Autodesk Inventor part; units mm, degrees
ref_plane "YZ Plane" through (0, 0, 0) normal (1, 0, 0) x (0, 1, 0)
ref_plane "XZ Plane" through (0, 0, 0) normal (0, 1, 0) x (-1, 0, 0)
ref_plane "XY Plane" through (0, 0, 0) normal (0, 0, 1) x (1, 0, 0)
sketch "Sketch1" plane through (0, 0, 0) normal (0, 1, 0) x (-1, 0, 0)
  circle A0 centre (0, 0) radius 3.75
  circle A1 centre (0, 0) radius 6
  dimension "d0" = 7.5
  dimension "d1" = 12
extrude "Extrusion1" add sketch "Sketch1" along normal blind 50 contours A0 | A1
extrude "Extrusion2" add sketch "Sketch1" against normal blind 2 contours A0
sketch "Sketch2" plane through (0, -2, 0) normal (0, -1, 0) x (1, 0, 0)
  circle A0 centre (0, 0) radius 1.85
  dimension "d6" = 3.7
extrude "Extrusion3" cut sketch "Sketch2" against normal blind 600
sketch "Sketch3" plane through (0, 50, 0) normal (0, 1, 0) x (1, 0, 0)
  circle A0 centre (0, 0) radius 1.85
  circle A1 centre (0, 0) radius 3.75
  dimension "d9" = 7.5
extrude "Extrusion4" add sketch "Sketch3" along normal blind 2
properties part number "extendo1"
For this review, take the finished solid that the model builds, in its own axes (mm). A direction names the side the tool comes from. Coordinates: 2 decimals unless noted, no trailing zeros. Loops run counter-clockwise (first coordinate to the right, second up) from the corner with the lowest first, then second, coordinate; pieces in that order, holes last. Notation, with made-up numbers: (64.25, -36) - (76.25, -36) arc R18 ccw to (76.25, -26) - close; hole circle Ø4 at (80.25, 87). An arc over 180 degrees is marked (long way). Use a Markdown table: item, result. Add a question column.
Item 1: Mouldability with a two-part tool opening along X and no side actions: class faces 4 (the face through (3.746, -0.986, 0.165)), 5 (the face through (1, 52, -2)), 6 (the face through (-0.401, 24.622, -1.806)) as pulls with the +X half, pulls with the -X half, needs draft (parallel to the pull), parting line crosses it, or undercut.
Item 2: We need section A-A (x = 0). Give the boundary of the cut face in (y, z), and give its area (3 significant figures).
Item 3: Insertion check: pin 1 Ø1.5 at (x, y) = (2, 39.5) entering from -Z; pin 2 Ø4 at (x, z) = (4.5, -3) entering from -Y; pin 3 Ø1 at (x, y) = (-2.5, 44.5) entering from -Z. Each pin has a flat end and moves straight along its axis. Give the tip position at first contact, or say it passes through.
Item 4: We need section B-B (z = 0). Give the boundary of the cut face in (x, y).
Item 5: We need section D-D (x = 3). Give the boundary of the cut face in (y, z), and give its area (3 significant figures).
Item 6: For line 1 (Z direction, x = 0, y = 28.5); line 2 (X direction, y = 36, z = 1.25); line 3 (Y direction, x = 5, z = -2.5), list the stretches that pass through material, from the lowest coordinate up.
Item 7: Tool access review of faces 1 (the face through (3, 0, -3)), 2 (the face through (3, 50, -3)), 3 (the face through (-1, -2, 2)): name each direction out of +Z, -Z, +X, -X, +Y, -Y from which nothing blocks a thin tool from reaching the whole face with its end or side.
Item 8: We need section C-C (y = 22.5). Give the boundary of the cut face in (x, z).
Results list:
| question | item | result |
|---|---|---|
| 1 | face 4 | parting line crosses it |
| 1 | face 5 | needs draft |
| 1 | face 6 | undercut |
| 2 | outline | (-2, -3.75) - (0, -3.75) - (0, -6) - (50, -6) - (50, -3.75) - (52, -3.75) - (52, -1.85) - (-2, -1.85) - close; (-2, 1.85) - (52, 1.85) - (52, 3.75) - (50, 3.75) - (50, 6) - (0, 6) - (0, 3.75) - (-2, 3.75) - close |
| 2 | area | 430 mm^2 |
| 3 | pin 1 | stops at z = -5.87 |
| 3 | pin 2 | stops at y = -2 |
| 3 | pin 3 | stops at z = -5.66 |
| 4 | outline | (-6, 0) - (-3.75, 0) - (-3.75, -2) - (-1.85, -2) - (-1.85, 52) - (-3.75, 52) - (-3.75, 50) - (-6, 50) - close; (1.85, -2) - (3.75, -2) - (3.75, 0) - (6, 0) - (6, 50) - (3.75, 50) - (3.75, 52) - (1.85, 52) - close |
| 5 | outline | (-2, -2.25) - (0, -2.25) - (0, -5.2) - (50, -5.2) - (50, -2.25) - (52, -2.25) - (52, 2.25) - (50, 2.25) - (50, 5.2) - (0, 5.2) - (0, 2.25) - (-2, 2.25) - close |
| 5 | area | 538 mm^2 |
| 6 | line 1 | z = -6 to -1.85, 1.85 to 6 |
| 6 | line 2 | x = -5.87 to -1.36, 1.36 to 5.87 |
| 6 | line 3 | y = 0 to 50 |
| 7 | face 1 | -Y |
| 7 | face 2 | +Y |
| 7 | face 3 | +Z, -Z, +X, -X, -Y |
| 8 | outline | circle Ø12 at (0, 0); hole circle Ø3.7 at (0, 0) |
